from build123d import *

# Parameters (mm, degrees)
F2_R     = 9.4996
F3_R     = 0.5
F4_DEPTH = 58


with BuildPart() as f1:
    # F0 (on Front) → F1 (revolve)
    with BuildSketch(Plane.XZ):
        with BuildLine():
            Line((0, 4.25), (0, 0))
            Line((0, 0), (8, 0))
            Line((8, 0), (64.008, 0))
            Line((64.008, 0), (64.008, 9.4996))
            Line((64.008, 9.4996), (47.55421, 9.4996))
            Line((47.55421, 9.4996), (32.004, 9.4996))
            Line((32.004, 9.4996), (19.776605, 9.4996))
            ThreePointArc((19.776605, 9.4996), (13.453427, 7.850371), (8, 4.25))
            Line((8, 4.25), (0, 4.25))
        make_face()
    revolve(axis=Axis((32.004, 0, 0), (1, 0, 0)))

    # F2
    f2_edges = [f1.edges().sort_by_distance(p)[0] for p in [
        (64.008, 0, -9.4996),
    ]]
    fillet(f2_edges, radius=F2_R)

    # F3 (on face) → F4 (cut)
    with BuildSketch(Plane(origin=(0, 0, 0), x_dir=(0, -1, 0), z_dir=(-1, 0, 0))):
        Circle(F3_R)
    extrude(amount=-F4_DEPTH, mode=Mode.SUBTRACT)


solid = f1.part
CAD build for the part. Positions are in the model's coordinates, mm. A direction names the side the tool comes from. Round coordinates to 2 decimals unless told otherwise and drop trailing zeros. Write each loop counter-clockwise with the first axis right and the second up, starting at its lowest first coordinate (ties: lowest second). Pieces come first, ordered by that corner, then holes.
(1) Drop flat-ended pins along their axis: P1, Ø1, axis at x = 50.5, y = 6.5, coming from the +Z side; P2, Ø5, axis at x = 50.5, z = 4.5, coming from the +Y side; P3, Ø1, axis at y = -3, z = 0.5, coming from the +X side; P4, Ø5, axis at y = -4.5, z = 3.5, coming from the -X side. Give the stop position or say it passes through.
(2) Slice it at A-A, the plane x = 30. Write the cut outline in (y, z).
(3) 3-axis set-ups, long thin cutter, end or side, ignore diameter. For faces 1 (the face through (3.944, -3.584, 2.285)), 2 (the face through (36.9, -6.42, -7)): which of +Z, -Z, +X, -X, +Y, -Y reach the whole face in a straight line?
(4) Probe line 1 along Z through (x, y) = (32, 0); line 2 along X through (y, z) = (0, 0.25); line 3 along Z through (x, y) = (56, -0.25). List the from-to ranges inside material, lowest first.
(5) Slice it at B-B, the plane x = 59. Write the cut outline in (y, z).
From the geometry:
1. P1: stops at z = 7.36
1. P2: stops at y = 9.29
1. P3: stops at x = 63.66
1. P4: stops at x = 0
2. outline: circle Ø19 at (0, 0); hole circle Ø1 at (0, 0)
3. face 1: -X
3. face 2: +X, -X
4. line 1: z = -9.5 to -0.5, 0.5 to 9.5
4. line 2: x = 58 to 64
4. line 3: z = -9.38 to -0.43, 0.43 to 9.38
5. outline: circle Ø16.74 at (0, 0)
